Input: part model. Units: mm. Frame: model coordinates. A direction names the side the tool comes from. Round coordinates to 2 decimals unless told otherwise and drop trailing zeros. Order: outer loops, then holes, each group sorted by start corner. A loop starts at its lowest first (then second) coordinate and runs counter-clockwise, first axis right, second up.
Item 1: Cut plane A-A on x = -20. Output: boundary loops of the cut face in (y, z).
Item 2: Reachability of faces 1 (the flat face through (38, -4.049, -66)), 2 (the flat face through (-24.049, 18, -66)), 3 (the flat face through (38.222, 14, -66)) from +Z, -Z, +X, -X, +Y, -Y: full face, straight path, thin tool, end or side. Return the list, or none.
Item 3: Cut plane C-C on x = -7.5. Output: boundary loops of the cut face in (y, z), then the cut area to 3 significant figures.
Item 4: Cut plane B-B on z = -107.5. Give the number of separate pieces and of enclosed holes in the cut face, then the cut area to 3 significant figures.
Item 5: First-contact query: pin 1 (8 mm diameter, centred on y = -1, z = -110, fed in from +X). Flat tip, straight axial feed; report the tip coordinate or a pass-through.
Item 6: Cut plane D-D on x = 2. Output: boundary loops of the cut face in (y, z), then the cut area to 3 significant figures.
Item 7: Mould query, pull axis X, two halves, no side actions, for faces 4 (the flat face through (20, -7.681, -66)), 5 (the flat face through (40, -10, -66)), 6 (the flat face through (9, -10, 0)). Classes: released by +X, released by -X, zero draft, split by the parting line, or undercut.
Item 8: Line query: L1, parallel to X at y = 0, z = -83; L2, parallel to X at y = 0, z = -16; L3, parallel to Y at x = -20, z = -79. Output: solid intervals per line, ascending.
```python
from build123d import *

# Parameters (mm, degrees)
SKETCH2_R                            = 3.35
F_40_SERIES_TS40_80LM_650037_1_DEPTH = 130
M8X1_25_TAPPED_HOLE1_D               = 6.8
M8X1_25_TAPPED_HOLE1_DEPTH           = 30
M8X1_25_TAPPED_HOLE1_TIP             = 2.042926105


with BuildPart() as part:
    # Sketch2 → 40 series TS40-80LM-650037(1) (new body)
    with BuildSketch(Plane(origin=(0, 0, -130), x_dir=(0, 1, 0), z_dir=(0, 0, 1))):
        with BuildLine():
            Line((0, -27.681), (-5.525738531, -27.681))
            Line((-5.525738531, -27.681), (-11.176, -33.331261469))
            Line((-11.176, -33.331261469), (-11.176, -36.6218))
            Line((-11.176, -36.6218), (-7.6835, -36.6218))
            Line((-7.6835, -36.6218), (-7.6835, -35.2248))
            Line((-7.6835, -35.2248), (-4.0488, -35.2248))
            Line((-4.0488, -35.2248), (-4.0488, -40))
            Line((-4.0488, -40), (-17, -40))
            ThreePointArc((-17, -40), (-19.121320344, -39.121320344), (-20, -37))
            Line((-20, -37), (-20, -24.0488))
            Line((-20, -24.0488), (-15.2248, -24.0488))
            Line((-15.2248, -24.0488), (-15.2248, -27.6835))
            Line((-15.2248, -27.6835), (-16.6218, -27.6835))
            Line((-16.6218, -27.6835), (-16.6218, -31.176))
            Line((-16.6218, -31.176), (-13.331261469, -31.176))
            Line((-13.331261469, -31.176), (-7.681, -25.525738531))
            Line((-7.681, -25.525738531), (-7.681, -20))
            Line((-7.681, -20), (-7.681, -14.474261469))
            Line((-7.681, -14.474261469), (-13.331261469, -8.824))
            Line((-13.331261469, -8.824), (-16.6218, -8.824))
            Line((-16.6218, -8.824), (-16.6218, -12.3165))
            Line((-16.6218, -12.3165), (-15.2248, -12.3165))
            Line((-15.2248, -12.3165), (-15.2248, -15.9512))
            Line((-15.2248, -15.9512), (-20, -15.9512))
            Line((-20, -15.9512), (-20, 15.9512))
            Line((-20, 15.9512), (-15.2248, 15.9512))
            Line((-15.2248, 15.9512), (-15.2248, 12.3165))
            Line((-15.2248, 12.3165), (-16.6218, 12.3165))
            Line((-16.6218, 12.3165), (-16.6218, 8.824))
            Line((-16.6218, 8.824), (-13.331261469, 8.824))
            Line((-13.331261469, 8.824), (-7.681, 14.474261469))
            Line((-7.681, 14.474261469), (-7.681, 25.525738531))
            Line((-7.681, 25.525738531), (-13.331261469, 31.176))
            Line((-13.331261469, 31.176), (-16.6218, 31.176))
            Line((-16.6218, 31.176), (-16.6218, 27.6835))
            Line((-16.6218, 27.6835), (-15.2248, 27.6835))
            Line((-15.2248, 27.6835), (-15.2248, 24.0488))
            Line((-15.2248, 24.0488), (-20, 24.0488))
            Line((-20, 24.0488), (-20, 37))
            ThreePointArc((-20, 37), (-19.121320344, 39.121320344), (-17, 40))
            Line((-17, 40), (-4.0488, 40))
            Line((-4.0488, 40), (-4.0488, 35.2248))
            Line((-4.0488, 35.2248), (-7.6835, 35.2248))
            Line((-7.6835, 35.2248), (-7.6835, 36.6218))
            Line((-7.6835, 36.6218), (-11.176, 36.6218))
            Line((-11.176, 36.6218), (-11.176, 33.331261469))
            Line((-11.176, 33.331261469), (-5.525738531, 27.681))
            Line((-5.525738531, 27.681), (0, 27.681))
            Line((0, 27.681), (5.525738531, 27.681))
            Line((5.525738531, 27.681), (11.176, 33.331261469))
            Line((11.176, 33.331261469), (11.176, 36.6218))
            Line((11.176, 36.6218), (7.6835, 36.6218))
            Line((7.6835, 36.6218), (7.6835, 35.2248))
            Line((7.6835, 35.2248), (4.0488, 35.2248))
            Line((4.0488, 35.2248), (4.0488, 40))
            Line((4.0488, 40), (17, 40))
            ThreePointArc((17, 40), (19.121320344, 39.121320344), (20, 37))
            Line((20, 37), (20, 24.0488))
            Line((20, 24.0488), (15.2248, 24.0488))
            Line((15.2248, 24.0488), (15.2248, 27.6835))
            Line((15.2248, 27.6835), (16.6218, 27.6835))
            Line((16.6218, 27.6835), (16.6218, 31.176))
            Line((16.6218, 31.176), (13.331261469, 31.176))
            Line((13.331261469, 31.176), (7.681, 25.525738531))
            Line((7.681, 25.525738531), (7.681, 20))
            Line((7.681, 20), (7.681, 14.474261469))
            Line((7.681, 14.474261469), (13.331261469, 8.824))
            Line((13.331261469, 8.824), (16.6218, 8.824))
            Line((16.6218, 8.824), (16.6218, 12.3165))
            Line((16.6218, 12.3165), (15.2248, 12.3165))
            Line((15.2248, 12.3165), (15.2248, 15.9512))
            Line((15.2248, 15.9512), (20, 15.9512))
            Line((20, 15.9512), (20, -15.9512))
            Line((20, -15.9512), (15.2248, -15.9512))
            Line((15.2248, -15.9512), (15.2248, -12.3165))
            Line((15.2248, -12.3165), (16.6218, -12.3165))
            Line((16.6218, -12.3165), (16.6218, -8.824))
            Line((16.6218, -8.824), (13.331261469, -8.824))
            Line((13.331261469, -8.824), (7.681, -14.474261469))
            Line((7.681, -14.474261469), (7.681, -20))
            Line((7.681, -20), (7.681, -25.525738531))
            Line((7.681, -25.525738531), (13.331261469, -31.176))
            Line((13.331261469, -31.176), (16.6218, -31.176))
            Line((16.6218, -31.176), (16.6218, -27.6835))
            Line((16.6218, -27.6835), (15.2248, -27.6835))
            Line((15.2248, -27.6835), (15.2248, -24.0488))
            Line((15.2248, -24.0488), (20, -24.0488))
            Line((20, -24.0488), (20, -37))
            ThreePointArc((20, -37), (19.121320344, -39.121320344), (17, -40))
            Line((17, -40), (4.0488, -40))
            Line((4.0488, -40), (4.0488, -35.2248))
            Line((4.0488, -35.2248), (7.6835, -35.2248))
            Line((7.6835, -35.2248), (7.6835, -36.6218))
            Line((7.6835, -36.6218), (11.176, -36.6218))
            Line((11.176, -36.6218), (11.176, -33.331261469))
            Line((11.176, -33.331261469), (5.525738531, -27.681))
            Line((5.525738531, -27.681), (0, -27.681))
        make_face()
        with Locations((0, -20)):
            Circle(SKETCH2_R, mode=Mode.SUBTRACT)
        with Locations((0, 20)):
            Circle(SKETCH2_R, mode=Mode.SUBTRACT)
        Polygon((-5.525738531, 12.319), (-17.844738531, 0), (-5.525738531, -12.319), (0, -12.319), (5.525738531, -12.319), (17.844738531, 0), (5.525738531, 12.319), (0, 12.319), align=None, mode=Mode.SUBTRACT)
        with BuildLine():
            Line((12.8372, 38.222), (12.8372, 32.8372))
            Line((12.8372, 32.8372), (18.222, 32.8372))
            Line((18.222, 32.8372), (18.222, 35.428))
            ThreePointArc((18.222, 35.428), (17.403656347, 37.403656347), (15.428, 38.222))
            Line((15.428, 38.222), (12.8372, 38.222))
        make_face(mode=Mode.SUBTRACT)
        with BuildLine():
            Line((12.8372, -32.8372), (18.222, -32.8372))
            Line((18.222, -32.8372), (18.222, -35.428))
            ThreePointArc((18.222, -35.428), (17.403656347, -37.403656347), (15.428, -38.222))
            Line((15.428, -38.222), (12.8372, -38.222))
            Line((12.8372, -38.222), (12.8372, -32.8372))
        make_face(mode=Mode.SUBTRACT)
        with BuildLine():
            Line((-12.8372, -38.222), (-12.8372, -32.8372))
            Line((-12.8372, -32.8372), (-18.222, -32.8372))
            Line((-18.222, -32.8372), (-18.222, -35.428))
            ThreePointArc((-18.222, -35.428), (-17.403656347, -37.403656347), (-15.428, -38.222))
            Line((-15.428, -38.222), (-12.8372, -38.222))
        make_face(mode=Mode.SUBTRACT)
        with BuildLine():
            Line((-18.222, 35.428), (-18.222, 32.8372))
            Line((-18.222, 32.8372), (-12.8372, 32.8372))
            Line((-12.8372, 32.8372), (-12.8372, 38.222))
            Line((-12.8372, 38.222), (-15.428, 38.222))
            ThreePointArc((-15.428, 38.222), (-17.403656347, 37.403656347), (-18.222, 35.428))
        make_face(mode=Mode.SUBTRACT)
    extrude(amount=F_40_SERIES_TS40_80LM_650037_1_DEPTH)

    # M8x1.25 Tapped Hole1
    with Locations(Plane.XY):
        with Locations((-20, 0), (20, 0)):
            Hole(M8X1_25_TAPPED_HOLE1_D / 2, depth=M8X1_25_TAPPED_HOLE1_DEPTH)
            with Locations((0, 0, -(M8X1_25_TAPPED_HOLE1_DEPTH + M8X1_25_TAPPED_HOLE1_TIP / 2))):  # 118° drill point
                Cone(0, M8X1_25_TAPPED_HOLE1_D / 2, M8X1_25_TAPPED_HOLE1_TIP, mode=Mode.SUBTRACT)


solid = part.part
```
From the geometry:
1. outline: (-7.68, -130) - (-3.35, -130) - (-3.35, -30.03) - (-3.4, -30) - (-3.4, 0) - (-7.68, 0) - close; (3.35, -130) - (7.68, -130) - (7.68, 0) - (3.4, 0) - (3.4, -30) - (3.35, -30.03) - close
2. face 1: +Z, -Z, +X
2. face 2: +Z, -Z, +Y
2. face 3: +Z, -Z
3. outline: (-20, -130) - (-10.34, -130) - (-10.34, 0) - (-20, 0) - close; (10.34, -130) - (20, -130) - (20, 0) - (10.34, 0) - close
3. area: 2,510 mm2
4. separate pieces: 1
4. enclosed holes: 7
4. area: 1,330 mm2
5. pin 1: stops at x = 40
6. outline: (-20, -130) - (-15.84, -130) - (-15.84, 0) - (-20, 0) - close; (15.84, -130) - (20, -130) - (20, 0) - (15.84, 0) - close
6. area: 1,080 mm2
7. face 4: undercut
7. face 5: released by +X
7. face 6: zero draft
8. L1: x = -27.68 to -23.35, -16.65 to -12.32, 12.32 to 16.65, 23.35 to 27.68
8. L2: x = -27.68 to -23.4, -16.6 to -12.32, 12.32 to 16.6, 23.4 to 27.68
8. L3: y = -7.68 to -3.35, 3.35 to 7.68
